Here's how the part is built. I have some questions about the finished solid (model axes, mm). Face numbers are marked on the shaded views. A direction names the side the tool comes from. Give positions to 0.01 mm unless a question says otherwise; leave off trailing zeros. Write each loop counter-clockwise with the first axis right and the second up, starting at its lowest first coordinate (ties: lowest second). Pieces come first, ordered by that corner, then holes. Notation, with made-up numbers: (25, 85) -> (51, 85) arc R17 cw to (51, 95) -> close; hole circle Ø9 at (52.5, -22). An arc over 180 degrees is marked (long way). Answer as CSV lines item,"result". Start each with the question number.
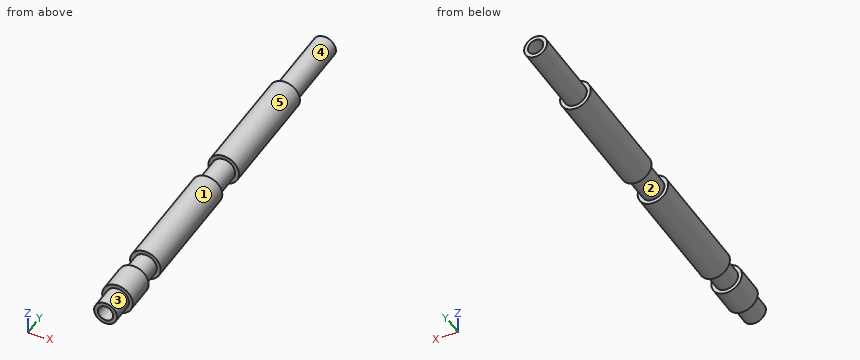
from build123d import *

# Parameters (mm, degrees)
SKETCH_1_R      = 2
SKETCH_1_R_2    = 1
EXTRUDE_1_DEPTH = 55
SKETCH_2_W      = 0.5
SKETCH_2_H      = 3
SKETCH_2_H_2    = 10
SKETCH_4_W      = 0.5
SKETCH_4_H      = 4.2


with BuildPart() as part:
    # Эскиз1 → Бобышка-Вытянуть1 (new body)
    with BuildSketch(Plane(origin=(0, 0, 0), x_dir=(1, 0, 0), z_dir=(0, 1, 0))):
        Circle(SKETCH_1_R)
        Circle(SKETCH_1_R_2, mode=Mode.SUBTRACT)
    extrude(amount=EXTRUDE_1_DEPTH)

    # Эскиз2 → Вырез-Повернуть1 (revolve, cut)
    with BuildSketch(Plane.XY):
        with Locations((1.75, 1.5)):
            Rectangle(SKETCH_2_W, SKETCH_2_H)
        with Locations((1.75, 8.5)):
            Rectangle(SKETCH_2_W, SKETCH_2_H)
        with Locations((1.75, 50)):
            Rectangle(SKETCH_2_W, SKETCH_2_H_2)
    revolve(axis=Axis((0, 0, 0), (0, 1, 0)), mode=Mode.SUBTRACT)

    # Эскиз4 → Вырез-Повернуть2 (revolve, cut)
    with BuildSketch(Plane.XY):
        with Locations((-1.75, 27.6)):
            Rectangle(SKETCH_4_W, SKETCH_4_H)
    revolve(axis=Axis((0, 0, 0), (0, 1, 0)), mode=Mode.SUBTRACT)


solid = part.part
Item 1: If I drill on line 1 (Y direction, x = -1.2, z = -1.4); line 2 (X direction, y = 34.5, z = 0), over which ranges is the centre line in solid material (lowest first)? Write a range as [from, to].
Item 2: We'd pull the mould along Y, two halves only. Please class the marked faces 1 and 2: released by +Y, released by -Y, zero draft, split by the parting line, or undercut.
Item 3: If we section it at C-C (y = 12.5): Please give me the cut outline in (x, z).
Item 4: I'm going to push flat-ended pins straight in: pin 1 (1.5 mm diameter, centred on y = 10.5, z = 1.5, fed in from -X); pin 2 (1 mm diameter, centred on x = -0.5, y = 13.5, fed in from -Z). Where does each tip first touch, or does it pass through?
Item 5: For the marked faces 3, 4 and 5, which set-ups out of +Z, -Z, +X, -X, +Y, -Y let a thin tool reach every point of the face, with its end or its side?
Final values:
1,line 1,"[3, 7], [10, 25.5], [29.7, 45]"
1,line 2,"[-2, -1], [1, 2]"
2,face 1,"zero draft"
2,face 2,"undercut"
3,outline,"circle Ø4 at (0, 0); hole circle Ø2 at (0, 0)"
4,pin 1,"x = -1.85"
4,pin 2,"z = -2"
5,face 3,"-Y"
5,face 4,"+Y"
5,face 5,"+Y, -Y"
